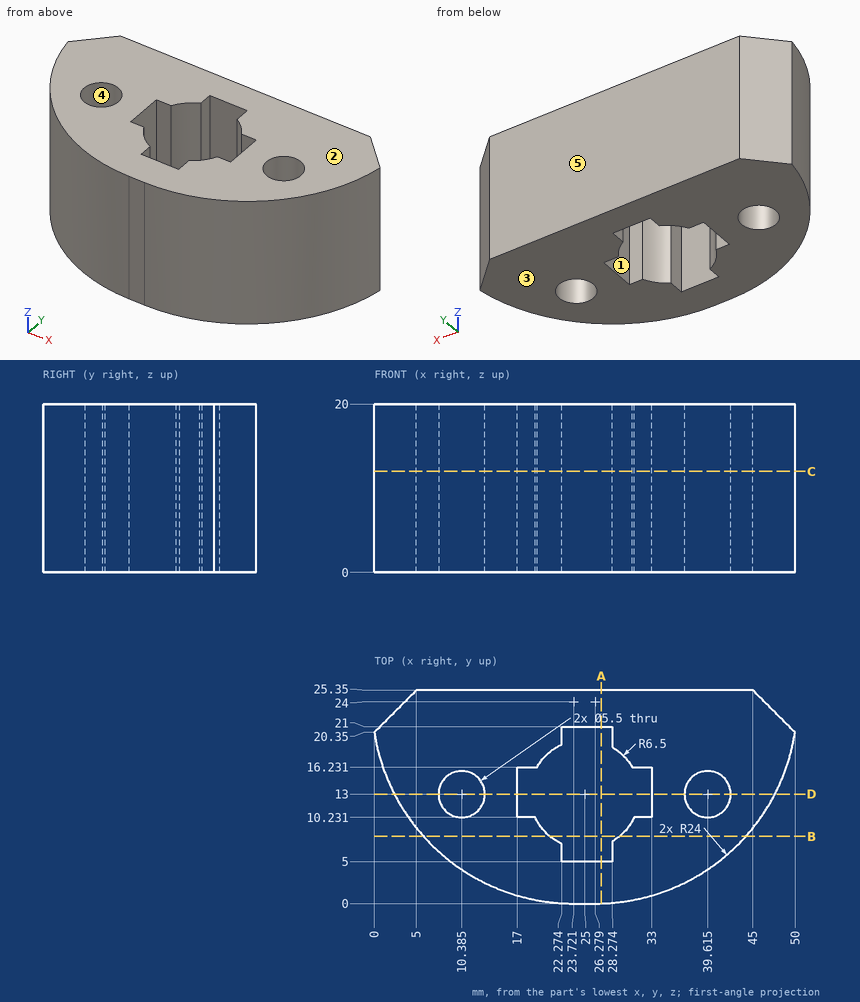
Study the drawing (mm; zero at the part's minimum x, y, z) and answer. A direction names the side the tool comes from. Give positions to 0.01 mm unless a question says otherwise; leave off trailing zeros. Loops run counter-clockwise (first coordinate to the right, second up) from the corner with the lowest first, then second, coordinate; pieces in that order, holes last. Notation, with made-up numbers: (-3.5, 77) - (18.5, 77) arc R9 cw to (18.5, 86) - close; hole circle Ø4 at (25, 82). An arc over 180 degrees is marked (long way). Answer as CSV lines item,"result". Start each with the question number.
1) Which of the six approach directions +Z, -Z, +X, -X, +Y, -Y give full straight-line access (tool end or side, diameter ignored) to the marked faces 1 and 2?
2) Straight lines are drawn through the part: L1, parallel to X at y = 11, z = 11 (1 decimal); L2, parallel to X at y = 15.5, z = 3 (1 decimal); L3, parallel to Y at x = 23, z = 4.25. For each, find the intervals that lie inside material, in ascending order. Write a range as from..to.
3) Find section B-B (y = 8). Write down the section's boundary in (x, z).
4) Find section C-C (z = 12). State how many separate pieces and enclosed holes the cut face has, then the cut area to 3 significant figures.
5) Find section D-D (y = 13). Write down the section's boundary in (x, z) (1 decimal).
6) Find section A-A (x = 27). Write down the section's boundary in (y, z).
7) Determine the mould class of the marked faces 3, 4 and 5 for opening direction Y: released by +Y, released by -Y, zero draft, split by the parting line, or undercut.
8) Each of these flat-tipped pins is pushed along its axis until it touches: pin 1 Ø5 at (y, z) = (13.5, 11) entering from -X; pin 2 Ø0.6 at (y, z) = (20, 14) entering from +X; pin 3 Ø1 at (x, z) = (15.5, 5) entering from -Y. Where does it stop, or does it pass through?
Findings below:
1,face 1,"+Z, -Z"
1,face 2,"+Z, +X, -X, +Y, -Y"
2,L1,"3.5..8.5, 12.3..17, 33..37.7, 41.5..46.5"
2,L2,"1.3..9.2, 11.5..17, 33..38.5, 40.8..48.7"
2,L3,"0.01..5, 21..25.35"
3,outline,"(5.83, 0) - (20.85, 0) - (20.85, 20) - (5.83, 20) - close; (29.15, 0) - (44.17, 0) - (44.17, 20) - (29.15, 20) - close"
4,separate pieces,"1"
4,enclosed holes,"3"
4,area,"785 mm^2"
5,outline,"(2.4, 0) - (7.6, 0) - (7.6, 20) - (2.4, 20) - close; (13.1, 0) - (17, 0) - (17, 20) - (13.1, 20) - close; (33, 0) - (36.9, 0) - (36.9, 20) - (33, 20) - close; (42.4, 0) - (47.6, 0) - (47.6, 20) - (42.4, 20) - close"
6,outline,"(0.01, 0) - (5, 0) - (5, 20) - (0.01, 20) - close; (21, 0) - (25.35, 0) - (25.35, 20) - (21, 20) - close"
7,face 3,"zero draft"
7,face 4,"undercut"
7,face 5,"released by +Y"
8,pin 1,"x = 1.09"
8,pin 2,"x = 49.99"
8,pin 3,"y = 1.28"
